Can you work these out from the model? Positions are in its coordinate system, mm. A direction names the side the tool comes from. Give positions to 0.01 mm unless a question says otherwise; leave off trailing zeros. Loops run counter-clockwise (first coordinate to the right, second up) from the corner with the lowest first, then second, coordinate; pieces in that order, holes last. Notation, with made-up numbers: (52.5, 66) - (77.5, 66) arc R30 ccw to (77.5, 91) - close; hole circle Ø6 at (-17, 15). An arc over 180 degrees is marked (long way). Answer as a JSON object with one key per item and string values.
```python
from build123d import *

# Parameters (mm, degrees)
BOSS_EXTRUDE1_DEPTH = 80


with BuildPart() as part:
    # Sketch1 → Boss-Extrude1 (new body)
    with BuildSketch(Plane.XY.offset(80)):
        with BuildLine():
            Line((-22, 24.5), (-22, 22))
            Line((-22, 22), (0, 22))
            Line((0, 22), (0, 0))
            Line((0, 0), (2.5, 0))
            ThreePointArc((2.5, 0), (7.803300859, 2.196699141), (10, 7.5))
            Line((10, 7.5), (10, 24.5))
            ThreePointArc((10, 24.5), (7.803300859, 29.803300859), (2.5, 32))
            Line((2.5, 32), (-14.5, 32))
            ThreePointArc((-14.5, 32), (-19.803300859, 29.803300859), (-22, 24.5))
        make_face()
    extrude(amount=-BOSS_EXTRUDE1_DEPTH)


solid = part.part
```
1) Imagine slicing it at C-C on x = -7. Write out the boundary of the cut face in (y, z).
Check sheet entries:
{"outline": "(22, 0) - (32, 0) - (32, 80) - (22, 80) - close"}
2) Imagine slicing it at A-A on z = 10. Write out the boundary of the cut face in (x, y), and give its area (3 significant figures).
Check sheet entries:
{"outline": "(-22, 22) - (0, 22) - (0, 0) - (2.5, 0) arc R7.5 ccw to (10, 7.5) - (10, 24.5) arc R7.5 ccw to (2.5, 32) - (-14.5, 32) arc R7.5 ccw to (-22, 24.5) - close", "area": "504 mm2"}
3) Which directions (+Z, -Z, +X, -X, +Y, -Y) give clear straight access to the entire face, cutting with the end or side of a thin tool? Please do faces 1 (the flat face through (-11, 22, 41)), 2 (the flat face through (-22, 23, 41)).
Check sheet entries:
{"face 1": "+Z, -Z, -X, -Y", "face 2": "+Z, -Z, -X, +Y, -Y"}
4) Imagine slicing it at B-B on y = 10. Write out the boundary of the cut face in (x, z).
Check sheet entries:
{"outline": "(0, 0) - (10, 0) - (10, 80) - (0, 80) - close"}
5) I'm going to push flat-ended pins straight in: P1, Ø17.5, axis at y = 9.5, z = 23, coming from the -X side; P2, Ø1, axis at x = 5.5, z = 23, coming from the -Y side; P3, Ø5, axis at y = 4.5, z = 54, coming from the +X side. Where does each tip first touch, or does it pass through?
Check sheet entries:
{"P1": "x = 0", "P2": "y = 0.43", "P3": "x = 9.98"}
6) I need wall thicknesses on L1, parallel to Y at x = -9.5, z = 75.5; L2, parallel to X at y = 13, z = 34; L3, parallel to Y at x = 5, z = 25. Which ranges of each line are inside material? Lowest first, please.
Check sheet entries:
{"L1": "22 to 32", "L2": "0 to 10", "L3": "0.43 to 31.57"}
